Can you work these out from the model? Positions are in its coordinate system, mm. A direction names the side the tool comes from. Coordinates: 2 decimals unless noted, no trailing zeros. Order: outer loops, then holes, each group sorted by start corner. A loop starts at its lowest first (then second) coordinate and runs counter-clockwise, first axis right, second up. Notation, with made-up numbers: (-9.5, -11.5) -> (49.5, -11.5) arc R17 ccw to (49.5, 5.5) -> close; hole circle Ø8 at (27.25, -9.75). An arc over 180 degrees is marked (long way). Write item = value, one per line. Start each with the question number.
from build123d import *

# Parameters (mm, degrees)
F1_DEPTH = 1.5
F3_DEPTH = 25
F6_DEPTH = 1.5
F7_W     = 3
F7_H     = 5
F8_DEPTH = 5


with BuildPart() as f1:
    # F0 (on Top) → F1 (new body)
    with BuildSketch(Plane.XY):
        with BuildLine():
            ThreePointArc((0, 1), (0.292893, 0.292893), (1, 0))
            Line((1, 0), (27, 0))
            ThreePointArc((27, 0), (27.707107, 0.292893), (28, 1))
            Line((28, 1), (28, 24.6))
            ThreePointArc((28, 24.6), (27.707107, 25.307107), (27, 25.6))
            Line((27, 25.6), (1, 25.6))
            ThreePointArc((1, 25.6), (0.292893, 25.307107), (0, 24.6))
            Line((0, 24.6), (0, 1))
        make_face()
    extrude(amount=F1_DEPTH)

    # F2 (on face) → F3 (cut)
    with BuildSketch(Plane.XY.offset(1.5)):
        with BuildLine():
            Line((6.3, 17.5), (6.3, 20))
            ThreePointArc((6.3, 20), (4.3, 22), (2.3, 20))
            Line((2.3, 20), (2.3, 17.5))
            ThreePointArc((2.3, 17.5), (4.3, 15.5), (6.3, 17.5))
        make_face()
        with BuildLine():
            Line((6.3, 5.6), (6.3, 8.1))
            ThreePointArc((6.3, 8.1), (4.3, 10.1), (2.3, 8.1))
            Line((2.3, 8.1), (2.3, 5.6))
            ThreePointArc((2.3, 5.6), (4.3, 3.6), (6.3, 5.6))
        make_face()
        with BuildLine():
            Line((25.7, 5.6), (25.7, 8.1))
            ThreePointArc((25.7, 8.1), (23.7, 10.1), (21.7, 8.1))
            Line((21.7, 8.1), (21.7, 5.6))
            ThreePointArc((21.7, 5.6), (23.7, 3.6), (25.7, 5.6))
        make_face()
        with BuildLine():
            Line((25.7, 17.5), (25.7, 20))
            ThreePointArc((25.7, 20), (23.7, 22), (21.7, 20))
            Line((21.7, 20), (21.7, 17.5))
            ThreePointArc((21.7, 17.5), (23.7, 15.5), (25.7, 17.5))
        make_face()
    extrude(amount=-F3_DEPTH, mode=Mode.SUBTRACT)

    # F5 (on offset) → F6 (join, symmetric)
    with BuildSketch(Plane.YZ.offset(14)):
        with BuildLine():
            Line((-3, 11.5), (0, 1.5))
            Line((0, 1.5), (25.6, 1.5))
            Line((25.6, 1.5), (25.6, 25))
            Line((25.6, 25), (54.1, 25))
            Line((54.1, 25), (54.1, 32))
            Line((54.1, 32), (21, 32))
            Line((21, 32), (15, 26))
            Line((15, 26), (15, 59.25))
            ThreePointArc((15, 59.25), (14.414214, 60.664214), (13, 61.25))
            Line((13, 61.25), (7.5, 61.25))
            ThreePointArc((7.5, 61.25), (6.085786, 60.664214), (5.5, 59.25))
            Line((5.5, 59.25), (5.5, 20.75))
            Line((5.5, 20.75), (-3, 11.5))
        make_face()
    extrude(amount=F6_DEPTH, both=True)

    # F7 (on face) → F8 (join)
    with BuildSketch(Plane(origin=(0, 0, 25), x_dir=(1, 0, 0), z_dir=(0, 0, -1))):
        with Locations((14, -43.8)):
            Rectangle(F7_W, F7_H)
    extrude(amount=F8_DEPTH)


solid = f1.part
(1) Imagine slicing it at D-D (z = 4.5). Write out the boundary of the cut face in (x, y).
(2) For faces 1 (the face through (15.5, 19, 25)), 2 (the face through (14, 18, 29)), 3 (the face through (4.3, 10.1, 0.8)), 4 (the face through (14, 50, 25)), which set-ups out of +Z, -Z, +X, -X, +Y, -Y let a thin tool reach every point of the face, with its end or its side?
(3) Imagine slicing it at B-B (y = 50). Write out the boundary of the cut face in (x, z).
(4) Imagine slicing it at A-A (x = 4.3). Write out the boundary of the cut face in (y, z), plus the area to 3 significant figures.
(5) For P1, Ø0.9, axis at x = 13.5, y = 29.5, coming from the -Z side; P2, Ø1.5, axis at x = 13.5, z = 23.5, coming from the +Y side; P3, Ø2.5, axis at x = 14, z = 36, coming from the +Y side, each with a flat end and sliding along its axis, tell me the tip position at first contact or that it passes through.
(6) Imagine slicing it at C-C (x = 24.5). Write out the boundary of the cut face in (y, z).
(7) If I drill on L1, parallel to Z at x = 23.25, y = 13; L2, parallel to X at y = 25.5, z = 16.5; L3, parallel to Z at x = 15, y = 18, over which ranges is the centre line in solid material (lowest first)? Write a range as from..to.
(8) Thinking about a two-plate mould opening in Y: for faces 5 (the face through (14, 41.3, 23)), 6 (the face through (23.7, 10.1, 0.8)), 7 (the face through (14, 0, 1)), 8 (the face through (22, 13, 1.5)), which applies, +Y half, -Y half, draft (parallel to the pull), parting line (faces both ways), or undercut?
Result set:
q1.outline = (12.5, -0.9) -> (15.5, -0.9) -> (15.5, 25.6) -> (12.5, 25.6) -> close
q2.face_1 = +Z, +X, +Y, -Y
q2.face_2 = +Z, +X, -X
q2.face_3 = +Z, -Z
q2.face_4 = -Z, +X, -X, +Y
q3.outline = (12.5, 25) -> (15.5, 25) -> (15.5, 32) -> (12.5, 32) -> close
q4.outline = (0, 0) -> (3.6, 0) -> (3.6, 1.5) -> (0, 1.5) -> close; (10.1, 0) -> (15.5, 0) -> (15.5, 1.5) -> (10.1, 1.5) -> close; (22, 0) -> (25.6, 0) -> (25.6, 1.5) -> (22, 1.5) -> close
q4.area = 18.9 mm2
q5.P1 = 25
q5.P2 = 46.3
q5.P3 = 15
q6.outline = (0, 0) -> (3.77, 0) -> (3.77, 1.5) -> (0, 1.5) -> close; (9.93, 0) -> (15.67, 0) -> (15.67, 1.5) -> (9.93, 1.5) -> close; (21.83, 0) -> (25.6, 0) -> (25.6, 1.5) -> (21.83, 1.5) -> close
q7.L1 = 0..1.5
q7.L2 = 12.5..15.5
q7.L3 = 0..29
q8.face_5 = undercut
q8.face_6 = undercut
q8.face_7 = -Y half
q8.face_8 = draft
